Here's how the part is built. I have some questions about the finished solid (model axes, mm). Round coordinates to 2 decimals unless told otherwise and drop trailing zeros. Order: outer loops, then holes, each group sorted by start corner. A loop starts at its lowest first (then second) coordinate and runs counter-clockwise, first axis right, second up. Notation, with made-up numbers: (38, -36) -> (82, -36) arc R20 cw to (82, -27) -> close; hole circle Ø4 at (48.25, -4.75). An arc over 180 degrees is marked (long way). Use a Markdown table: item, result. Add a question column.
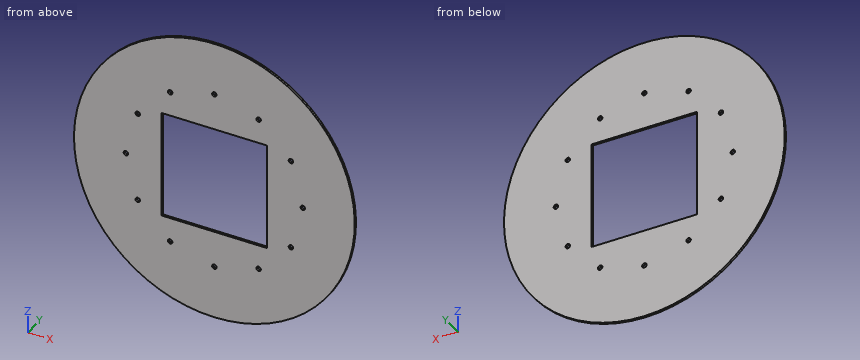
from build123d import *

# Parameters (mm, degrees)
SKETCH1_W           = 40
SKETCH1_H           = 1.57
BOSS_EXTRUDE1_START = -1.57
SKETCH2_R           = 60
SKETCH2_W           = 75
SKETCH2_H           = 75
BOSS_EXTRUDE1_DEPTH = 1.57
SKETCH3_R           = 1.6
CUT_EXTRUDE1_DEPTH  = 142.430070706
CIRPATTERN1_COUNT   = 12


with BuildPart() as part:
    # Sketch1 → Revolve1 (revolve)
    with BuildSketch(Plane.XY, mode=Mode.PRIVATE) as revolve1_sk:
        with Locations((-80, 0)):
            Rectangle(SKETCH1_W, SKETCH1_H)
    revolve(revolve1_sk.sketch.rotate(Axis((0, -200069.047495165, 0), (0, 1, 0)), 270), axis=Axis((0, -200069.047495165, 0), (0, 1, 0)))

    # Sketch2 → Boss-Extrude1 (add)
    with BuildSketch(Plane(origin=(0, 0.785, 0), x_dir=(1, 0, 0), z_dir=(0, 1, 0)).offset(BOSS_EXTRUDE1_START)):
        Circle(SKETCH2_R)
        Rectangle(SKETCH2_W, SKETCH2_H, mode=Mode.SUBTRACT)
    extrude(amount=BOSS_EXTRUDE1_DEPTH)

    # Sketch3 → Cut-Extrude1 (cut, through all)
    with BuildSketch(Plane(origin=(0, 0.785, 0), x_dir=(1, 0, 0), z_dir=(0, 1, 0))):
        with Locations(Location((0, 63, 0), (0, 0, 270))):
            Circle(SKETCH3_R)
    cut_extrude1 = extrude(amount=-CUT_EXTRUDE1_DEPTH, mode=Mode.SUBTRACT)

    # CirPattern1: Cut-Extrude1 ×12 about axis
    cirpattern1_axis = Axis((0, 0, 0), (0, 1, 0))
    for i in range(1, CIRPATTERN1_COUNT):
        add(cut_extrude1.rotate(cirpattern1_axis, i * 360 / CIRPATTERN1_COUNT), mode=Mode.SUBTRACT)


solid = part.part
(1) I want a section at D-D on z = 70. List the corners of the cut face in (x, y) for me (3 decimals), and give its area (3 significant figures).
(2) Please list where these lines run through material, in increasing order: probe 1 along Z at (x, y) = (31.5, 0.4); probe 2 along X at (y, z) = (-0.3, 53.5); probe 3 along Z at (x, y) = (-32.5, -0.3). Write a range as from..to.
(3) I want a section at A-A on z = 7.5. List the corners of the cut face in (x, y) for me (3 decimals), and give its area (3 significant figures).
(4) I want a section at B-B on x = -23.5. List the corners of the cut face in (y, z) for me (3 decimals).
(5) I want a section at C-C on x = 78. List the corners of the cut face in (y, z) for me (3 decimals), and give its area (3 significant figures).
(6) I'm going to push flat-ended pins straight in: P1, Ø0.5, axis at x = -10.5, y = 0, coming from the -Z side; P2, Ø0.5, axis at y = 0, z = -18, coming from the +X side. Where does each tip first touch, or does it pass through?
Output:
| question | item | result |
|---|---|---|
| 1 | outline | (-71.414, -0.785) -> (71.414, -0.785) -> (71.414, 0.785) -> (-71.414, 0.785) -> close |
| 1 | area | 224 mm² |
| 2 | probe 1 | -94.91..-56.16, -52.96..-37.5, 37.5..52.96, 56.16..94.91 |
| 2 | probe 2 | -84.49..-32.7, -30.3..30.3, 32.7..84.49 |
| 2 | probe 3 | -94.57..-55.81, -53.31..-37.5, 37.5..53.31, 55.81..94.57 |
| 3 | outline | (-99.718, -0.785) -> (-37.5, -0.785) -> (-37.5, 0.785) -> (-99.718, 0.785) -> close; (37.5, -0.785) -> (99.718, -0.785) -> (99.718, 0.785) -> (37.5, 0.785) -> close |
| 3 | area | 195 mm² |
| 4 | outline | (-0.785, -97.2) -> (0.785, -97.2) -> (0.785, -37.5) -> (-0.785, -37.5) -> close; (-0.785, 37.5) -> (0.785, 37.5) -> (0.785, 97.2) -> (-0.785, 97.2) -> close |
| 5 | outline | (-0.785, -62.578) -> (0.785, -62.578) -> (0.785, 62.578) -> (-0.785, 62.578) -> close |
| 5 | area | 196 mm² |
| 6 | P1 | z = -99.47 |
| 6 | P2 | x = 98.41 |
